Can you work these out from the model? Positions are in its coordinate system, mm. A direction names the side the tool comes from. Coordinates: 2 decimals unless noted, no trailing zeros. Order: outer loops, then holes, each group sorted by start corner. A loop starts at its lowest first (then second) coordinate and runs counter-clockwise, first axis right, second up. Notation, with made-up numbers: (49.5, 32.5) -> (86.5, 32.5) arc R16 ccw to (86.5, 43.5) -> close; hole circle Ø4 at (71.25, -18). An arc over 180 degrees is marked (long way). Answer as CSV lines item,"result".
from build123d import *

# Parameters (mm, degrees)
BOSS_EXTRUDE1_DEPTH = 20
SKETCH2_R           = 1.44
CUT_EXTRUDE1_DEPTH  = 21
DRAFT1_ANGLE        = 5
CUT_EXTRUDE2_DEPTH  = 5
DRAFT2_ANGLE        = 10


with BuildPart() as part:
    # Sketch1 → Boss-Extrude1 (new body)
    with BuildSketch(Plane(origin=(0, 0, 0), x_dir=(1, 0, 0), z_dir=(0, 1, 0))):
        Polygon((3.5, -5), (3.5, 5), (0, 6.5), (-3.5, 5), (-3.5, -5), (0, -6.5), align=None)
    extrude(amount=BOSS_EXTRUDE1_DEPTH)

    # Sketch2 → Cut-Extrude1 (cut, through all)
    with BuildSketch(Plane(origin=(0, 20, 0), x_dir=(1, 0, 0), z_dir=(0, 1, 0))):
        with Locations((0, 3)):
            Circle(SKETCH2_R)
        with Locations((0, -3)):
            Circle(SKETCH2_R)
    extrude(amount=-CUT_EXTRUDE1_DEPTH, mode=Mode.SUBTRACT)

    # Draft1
    draft1_faces = [part.faces().sort_by_distance(p)[0] for p in [
        (-3.5, 10, 0),
        (-1.75, 10, -5.75),
        (1.75, 10, -5.75),
        (3.5, 10, 0),
        (1.75, 10, 5.75),
        (-1.75, 10, 5.75),
    ]]
    draft(draft1_faces, Plane.ZX.offset(20), DRAFT1_ANGLE)

    # Sketch1<2> → Cut-Extrude2 (cut)
    with BuildSketch(Plane(origin=(0, 0, 0), x_dir=(1, 0, 0), z_dir=(0, 1, 0))):
        Polygon((3.5, -5), (3.5, 5), (0, 6.5), (-3.5, 5), (-3.5, -5), (0, -6.5), align=None)
    extrude(amount=CUT_EXTRUDE2_DEPTH, mode=Mode.SUBTRACT)

    # Draft2
    draft2_faces = [part.faces().sort_by_distance(p)[0] for p in [
        (-3.5, 2.5, 0),
        (-1.75, 2.5, 5.75),
        (1.75, 2.5, 5.75),
        (3.5, 2.5, 0),
        (1.75, 2.5, -5.75),
        (-1.75, 2.5, -5.75),
    ]]
    draft(draft2_faces, Plane(origin=(0, 5, 0), x_dir=(0, 0, -1), z_dir=(0, -1, 0)), DRAFT2_ANGLE)


solid = part.part
Q1. Imagine slicing it at A-A (x = 0.75). List the corners of the cut face in (y, z) for me.
Solution:
outline,"(0, -8.08) -> (20, -6.18) -> (20, -4.23) -> (5, -4.23) -> (5, -6.18) -> (0, -7.14) -> close; (0, 7.14) -> (5, 6.18) -> (5, 4.23) -> (20, 4.23) -> (20, 6.18) -> (0, 8.08) -> close; (5, -1.77) -> (20, -1.77) -> (20, 1.77) -> (5, 1.77) -> close"
Q2. Imagine slicing it at C-C (z = -1). List the corners of the cut face in (x, y) for me.
Solution:
outline,"(-5.25, 0) -> (-4.38, 0) -> (-3.5, 5) -> (3.5, 5) -> (4.38, 0) -> (5.25, 0) -> (3.5, 20) -> (-3.5, 20) -> close"
Q3. We'd pull the mould along X, two halves only. Please class faces 1 (the cylindrical face through (-0.187, 12.605, 1.572)), 2 (the flat face through (2.25, 9.86, 6.5)), 3 (the flat face through (-5, 0, 1)): pulls with the +X half, pulls with the -X half, needs draft (parallel to the pull), parting line crosses it, or undercut.
Solution:
face 1,"undercut"
face 2,"pulls with the +X half"
face 3,"needs draft"
Q4. If I drill on line 1 (Y direction, x = -0.5, z = -1); line 2 (X direction, y = 12.75, z = 3); line 3 (X direction, y = 16.25, z = -3), over which ranges is the centre line in solid material (lowest first)?
Solution:
line 1,"5 to 20"
line 2,"-4.13 to -1.44, 1.44 to 4.13"
line 3,"-3.83 to -1.44, 1.44 to 3.83"
Q5. Imagine slicing it at D-D (y = 1.5). List the corners of the cut face in (x, z) for me, and give its area (3 significant figures).
Solution:
outline,"(-5.12, -6.07) -> (0, -8.26) -> (5.12, -6.07) -> (5.12, 6.07) -> (0, 8.26) -> (-5.12, 6.07) -> close; hole (-4.12, -5.41) -> (0, -7.17) -> (4.12, -5.41) -> (4.12, 5.41) -> (0, 7.17) -> (-4.12, 5.41) -> close"
area,"43.1 mm2"
Q6. Which directions (+Z, -Z, +X, -X, +Y, -Y) give clear straight access to the entire face, cutting with the end or side of a thin tool? Please do faces 4 (the flat face through (4.387, 9.86, 0.086)), 5 (the flat face through (3.947, 2.465, 0.078)).
Solution:
face 4,"+Z, -Z, +X, +Y"
face 5,"-Y"
Q7. For P1, Ø10, axis at y = 18, z = -1.5, coming from the -X side; P2, Ø10, axis at y = 4, z = -5.5, coming from the -X side; P3, Ø3, axis at y = 16, z = 6, coming from the -X side; P4, Ø3, axis at y = 13, z = 1, coming from the -X side, each with a flat end and sliding along its axis, tell me the tip position at first contact or that it passes through.
Solution:
P1,"x = -4.11"
P2,"x = -5.25"
P3,"x = -3.97"
P4,"x = -4.24"
Q8. Imagine slicing it at B-B (z = -3.75). List the corners of the cut face in (x, y) for me.
Solution:
outline,"(-5.25, 0) -> (-4.38, 0) -> (-3.5, 5) -> (-1.23, 5) -> (-1.23, 20) -> (-3.5, 20) -> close; (1.23, 5) -> (3.5, 5) -> (4.38, 0) -> (5.25, 0) -> (3.5, 20) -> (1.23, 20) -> close"
